```python
from build123d import *

# Parameters (mm, degrees)
BOSS_EXTRUDE1_DEPTH     = 1
BOSS_EXTRUDE3_START     = 2
SKETCH2_R               = 2.1
BOSS_EXTRUDE3_DEPTH     = 2
CUT_EXTRUDE1_DEPTH      = 18.959719392
CUT_EXTRUDE1_DEPTH_BACK = 18.959719392
SKETCH3_R               = 1.325


with BuildPart() as part:
    # Sketch1 → Boss-Extrude1 (new, symmetric)
    with BuildSketch(Plane(origin=(0, 0, 0), x_dir=(1, 0, 0), z_dir=(0, 1, 0))):
        with BuildLine():
            ThreePointArc((-15.38117618, 2.1), (-17.48117618, 0), (-15.38117618, -2.1))
            Line((-15.38117618, -2.1), (-2.38117618, -2.7))
            ThreePointArc((-2.38117618, -2.7), (3.6, 0), (-2.38117618, 2.7))
            Line((-2.38117618, 2.7), (-15.38117618, 2.1))
        make_face()
    extrude(amount=BOSS_EXTRUDE1_DEPTH, both=True)

    # Sketch2 → Boss-Extrude3 (add)
    with BuildSketch(Plane(origin=(0, 1, 0), x_dir=(1, 0, 0), z_dir=(0, 1, 0)).offset(BOSS_EXTRUDE3_START)):
        with BuildLine():
            ThreePointArc((-2.38117618, 2.7), (-3.579161976, 0), (-2.38117618, -2.7))
            ThreePointArc((-2.38117618, -2.7), (3.6, 0), (-2.38117618, 2.7))
        make_face()
        with Locations(Location((0, 0, 0), (0, 0, 270))):
            Circle(SKETCH2_R, mode=Mode.SUBTRACT)
    extrude(amount=-BOSS_EXTRUDE3_DEPTH)

    # Sketch3 → Cut-Extrude1 (cut, two sides: drawn at the far end of the back side and taken through both)
    with BuildSketch(Plane(origin=(0, 1, 0), x_dir=(1, 0, 0), z_dir=(0, 1, 0)).offset(-CUT_EXTRUDE1_DEPTH_BACK)):
        with Locations(Location((0, 0, 0), (0, 0, 270))):
            Circle(SKETCH3_R)
    extrude(amount=CUT_EXTRUDE1_DEPTH + CUT_EXTRUDE1_DEPTH_BACK, mode=Mode.SUBTRACT)


solid = part.part
```
For this review, take the finished solid that the model builds, in its own axes (mm). A direction names the side the tool comes from. Round coordinates to 2 decimals unless told otherwise and drop trailing zeros. Write each loop counter-clockwise with the first axis right and the second up, starting at its lowest first coordinate (ties: lowest second). Pieces come first, ordered by that corner, then holes. Notation, with made-up numbers: M 32.25,-13 L 80.25,-13 A11 ccw 80.25,-1 Z; hole C 3,81 d2. An arc over 180 degrees is marked long. One line per item, written item: value. Start each with the question number.
(1) Machinability: for faces 4 (the cylindrical face through (-0.81, -0.01, -1.05)), 5 (the cylindrical face through (-3.58, 2.01, -0.04)), 6 (the flat face through (1.4, 1, -0.5)), which of the approach directions +Z, -Z, +X, -X, +Y, -Y give a long, thin tool a straight path to every point of the face, cutting with its end or side? Answer none if there is none.
(2) We need section C-C (y = 2.1). Give the boundary of the cut face in (x, z), and give its area (3 significant figures).
(3) We need section A-A (z = 0). Give the boundary of the cut face in (x, y) (3 decimals), and give its area (3 significant figures).
(4) We need section D-D (z = -1). Give the boundary of the cut face in (x, y).
(5) We need section B-B (x = 0). Give the boundary of the cut face in (y, z) (3 decimals), and give its area (3 significant figures).
(6) Insertion check: pin 1 (1 mm diameter, centred on y = 2.5, z = 0.5, fed in from +X); pin 2 (3.5 mm diameter, centred on x = 0, z = 0, fed in from +Y); pin 3 (1.5 mm diameter, centred on x = -13.5, y = 1.5, fed in from +Z). Each pin has a flat end and moves straight along its axis. Give the tip position at first contact, or say it passes through.
(7) The part is to be moulded in two halves that separate along Z. For faces 1 (the flat face through (-8.79, 0.014, -2.404)), 2 (the flat face through (2, 3, 2)), 3 (the cylindrical face through (0.631, 2.014, 2.003)), say which applies: released by +Z, released by -Z, zero draft, split by the parting line, or undercut.
(8) Wall thickness on line 1 (Z direction, x = 0, y = -0.55) (3 decimals); line 2 (Y direction, x = -12.5, z = -1.5); line 3 (X direction, y = 0.45, z = 0) (3 decimals): over which ranges is each line inside the solid? List them lowest first.
Result:
1. face 4: +Y, -Y
1. face 5: -X, +Y
1. face 6: +Y
2. outline: M -2.38,-2.7 A3.6 ccw long -2.38,2.7 A3.64 ccw Z; hole C 0,0 d4.2
2. area: 26.8 mm²
3. outline: M -17.481,-1 L -1.325,-1 L -1.325,1 L -2.1,1 L -2.1,3 L -3.579,3 L -3.579,1 L -17.481,1 Z; M 1.325,-1 L 3.6,-1 L 3.6,3 L 2.1,3 L 2.1,1 L 1.325,1 Z
3. area: 42.8 mm²
4. outline: M -17.23,-1 L -0.87,-1 L -0.87,1 L -1.85,1 L -1.85,3 L -3.44,3 L -3.44,1 L -17.23,1 Z; M 0.87,-1 L 3.46,-1 L 3.46,3 L 1.85,3 L 1.85,1 L 0.87,1 Z
5. outline: M -1,-3.6 L 3,-3.6 L 3,-2.1 L 1,-2.1 L 1,-1.325 L -1,-1.325 Z; M -1,1.325 L 1,1.325 L 1,2.1 L 3,2.1 L 3,3.6 L -1,3.6 Z
5. area: 15.1 mm²
6. pin 1: x = 3.6
6. pin 2: y = 1
6. pin 3: z = 2.21
7. face 1: released by -Z
7. face 2: zero draft
7. face 3: undercut
8. line 1: -3.6 to -1.325, 1.325 to 3.6
8. line 2: -1 to 1
8. line 3: -17.481 to -1.325, 1.325 to 3.6
